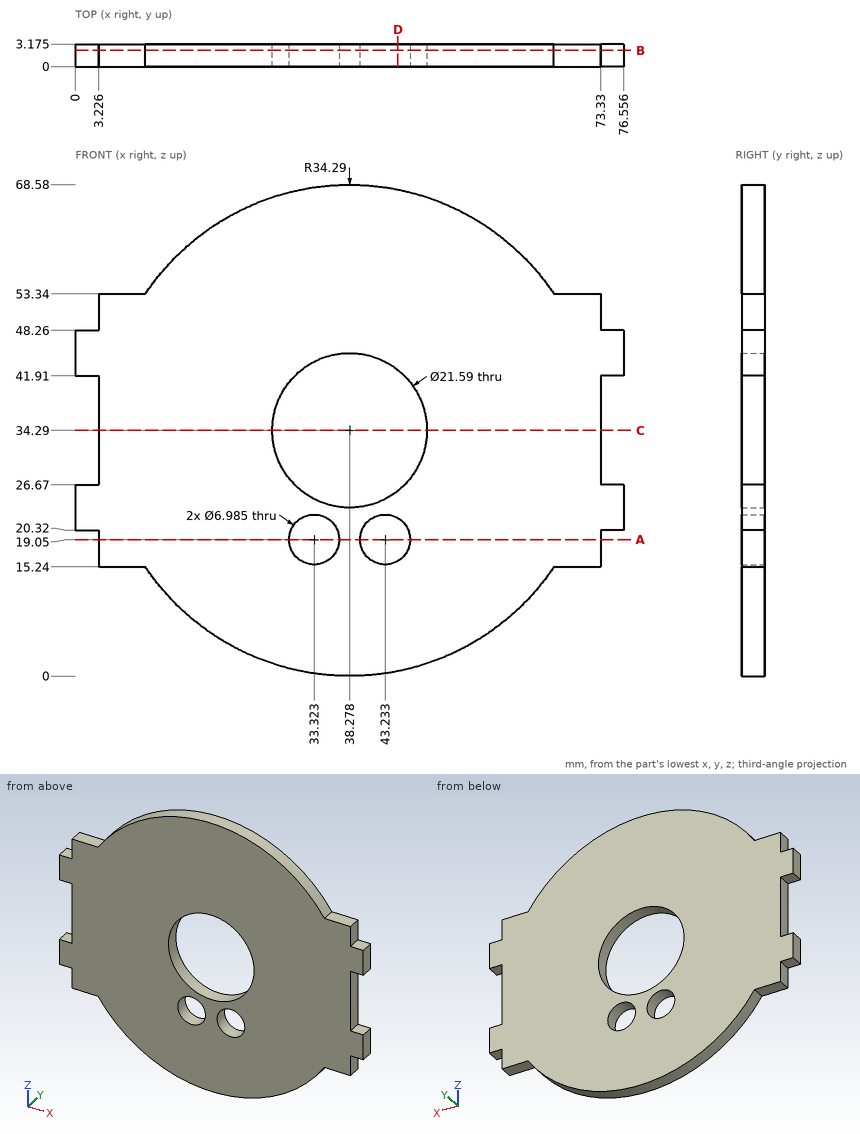
For this review, use the dimensioned drawing (mm, ordinates from the lowest corner) and the shaded views. Coordinates: 2 decimals unless noted, no trailing zeros. Order: outer loops, then holes, each group sorted by start corner. A loop starts at its lowest first (then second) coordinate and runs counter-clockwise, first axis right, second up. Notation, with made-up numbers: (56, 34) - (83, 34) arc R19 ccw to (83, 51) - close; hole circle Ø2 at (0.25, 24). An arc over 180 degrees is marked (long way). Answer in a Markdown table with one row per item.
(1) Wall thickness on line 1 along X through (y, z) = (0.8, 19.05) (1 decimal); line 2 along Z through (x, y) = (46, 2.2) (1 decimal); line 3 along Z through (x, y) = (35, 1.65) (1 decimal): over which ranges is each line inside the solid? List them lowest first. Write a range as from..to.
Checked values:
| item | result |
|---|---|
| line 1 | 3.2..29.8, 36.8..39.7, 46.7..73.3 |
| line 2 | 0.9..16.9, 21.2..26.7, 41.8..67.7 |
| line 3 | 0.2..16, 22.1..24, 44.6..68.4 |
(2) Consider section A-A on z = 19.05. State the section outline as (x, y) points (1 decimal).
Checked values:
| item | result |
|---|---|
| outline | (3.2, 0) - (29.8, 0) - (29.8, 3.2) - (3.2, 3.2) - close; (36.8, 0) - (39.7, 0) - (39.7, 3.2) - (36.8, 3.2) - close; (46.7, 0) - (73.3, 0) - (73.3, 3.2) - (46.7, 3.2) - close |
(3) Consider section D-D on x = 45. State the section outline as (y, z) points (1 decimal), plus the area to 3 significant figures.
Checked values:
| item | result |
|---|---|
| outline | (0, 0.7) - (3.2, 0.7) - (3.2, 16) - (0, 16) - close; (0, 22.1) - (3.2, 22.1) - (3.2, 25.8) - (0, 25.8) - close; (0, 42.7) - (3.2, 42.7) - (3.2, 67.9) - (0, 67.9) - close |
| area | 141 mm^2 |
(4) Consider section C-C on z = 34.29. State the section outline as (x, y) points (1 decimal), plus the area to 3 significant figures.
Checked values:
| item | result |
|---|---|
| outline | (3.2, 0) - (27.5, 0) - (27.5, 3.2) - (3.2, 3.2) - close; (49.1, 0) - (73.3, 0) - (73.3, 3.2) - (49.1, 3.2) - close |
| area | 154 mm^2 |
(5) Clearance check with flat-ended pins moving along their axes: pin 1 (1 mm diameter, centred on y = 1, z = 18.5, fed in from -X); pin 2 (1.6 mm diameter, centred on x = 2, y = 1, fed in from +Z); pin 3 (1 mm diameter, centred on y = 1.5, z = 51, fed in from +X). State where each tip first meets the part, or that it passes through.
Checked values:
| item | result |
|---|---|
| pin 1 | x = 3.23 |
| pin 2 | z = 48.26 |
| pin 3 | x = 73.33 |
(6) Consider section B-B on y = 2.3. Give the number of separate pieces and of enclosed holes in the cut face, plus the area to 3 significant figures.
Checked values:
| item | result |
|---|---|
| separate pieces | 1 |
| enclosed holes | 3 |
| area | 3,530 mm^2 |
